```python
from build123d import *

# Parameters (mm, degrees)
SKETCH1_R           = 31.5
SKETCH1_R_2         = 4
SKETCH1_R_3         = 5.1
SKETCH1_R_4         = 3.5
SKETCH1_R_5         = 3
SKETCH1_R_6         = 3.000009018
BOSS_EXTRUDE1_DEPTH = 10
SKETCH1_3_R         = 5.1
SKETCH1_3_R_2       = 3.5
SKETCH1_3_R_3       = 3
SKETCH1_3_R_4       = 2.5
SKETCH1_3_R_5       = 3.000009018
BOSS_EXTRUDE2_DEPTH = 2


with BuildPart() as part:
    # Sketch1 → Boss-Extrude1 (new body)
    with BuildSketch(Plane.XY):
        Circle(SKETCH1_R)
        Circle(SKETCH1_R_2, mode=Mode.SUBTRACT)
        with Locations((-19, 0)):
            Circle(SKETCH1_R_3, mode=Mode.SUBTRACT)
        with Locations((0, 19)):
            Circle(SKETCH1_R_3, mode=Mode.SUBTRACT)
        with Locations((-13.436536842, 13.433520674)):
            Circle(SKETCH1_R_4, mode=Mode.SUBTRACT)
        with Locations((19, 0)):
            Circle(SKETCH1_R_3, mode=Mode.SUBTRACT)
        with Locations((13.436536842, -13.433520674)):
            Circle(SKETCH1_R_4, mode=Mode.SUBTRACT)
        with Locations((0, -19)):
            Circle(SKETCH1_R_3, mode=Mode.SUBTRACT)
        with Locations((8.124653839, 25)):
            Circle(SKETCH1_R_5, mode=Mode.SUBTRACT)
        with Locations((-9.156294472, -23.262894737)):
            Circle(SKETCH1_R_6, mode=Mode.SUBTRACT)
    extrude(amount=BOSS_EXTRUDE1_DEPTH)

    # Sketch1_3 → Boss-Extrude2 (add)
    with BuildSketch(Plane.XY):
        with Locations((19, 0)):
            Circle(SKETCH1_3_R)
        with Locations((19, 0)):
            Circle(SKETCH1_3_R_2, mode=Mode.SUBTRACT)
        with Locations((0, 19)):
            Circle(SKETCH1_3_R)
        with Locations((0, 19)):
            Circle(SKETCH1_3_R_2, mode=Mode.SUBTRACT)
        with Locations((13.436536842, -13.433520674)):
            Circle(SKETCH1_3_R_2)
        with Locations((13.436536842, -13.433520674)):
            Circle(SKETCH1_3_R_3, mode=Mode.SUBTRACT)
        with Locations((-13.436536842, 13.433520674)):
            Circle(SKETCH1_3_R_2)
        with Locations((-13.436536842, 13.433520674)):
            Circle(SKETCH1_3_R_3, mode=Mode.SUBTRACT)
        with Locations((0, -19)):
            Circle(SKETCH1_3_R)
        with Locations((0, -19)):
            Circle(SKETCH1_3_R_2, mode=Mode.SUBTRACT)
        with Locations((-19, 0)):
            Circle(SKETCH1_3_R)
        with Locations((-19, 0)):
            Circle(SKETCH1_3_R_2, mode=Mode.SUBTRACT)
        with Locations((8.124653839, 25)):
            Circle(SKETCH1_3_R_3)
        with Locations((8.124653839, 25)):
            Circle(SKETCH1_3_R_4, mode=Mode.SUBTRACT)
        with Locations((-9.156294472, -23.262894737)):
            Circle(SKETCH1_3_R_5)
        with Locations((-9.156294472, -23.262894737)):
            Circle(SKETCH1_3_R_4, mode=Mode.SUBTRACT)
    extrude(amount=BOSS_EXTRUDE2_DEPTH)


solid = part.part
```
Could you check a few things on this model? Use its own coordinates, in mm. A direction names the side the tool comes from. Give positions to 0.01 mm unless a question says otherwise; leave off trailing zeros. Write each loop counter-clockwise with the first axis right and the second up, starting at its lowest first coordinate (ties: lowest second). Pieces come first, ordered by that corner, then holes. Notation, with made-up numbers: (9.25, 46.25) - (16.25, 46.25) arc R28 cw to (16.25, 84.25) - close; hole circle Ø8 at (-34.5, -39). An arc over 180 degrees is marked (long way). One line per item, written item: value. Start each with the question number.
Item 1: Imagine slicing it at B-B, the plane z = 9. Give the number of separate pieces and of enclosed holes in the cut face, and give its area (3 significant figures).
Item 2: I'm going to push flat-ended pins straight in: pin 1 (3 mm diameter, centred on x = 2.5, z = 4.5, fed in from +Y); pin 2 (3.5 mm diameter, centred on x = -14, y = 15, fed in from +Z); pin 3 (13.5 mm diameter, centred on x = 0, y = 19, fed in from -Z); pin 4 (1 mm diameter, centred on y = 25, z = 5, fed in from +X). Where does each tip first touch, or does it pass through?
Item 3: Which directions (+Z, -Z, +X, -X, +Y, -Y) give clear straight access to the entire face, cutting with the end or side of a thin tool? Please do faces 1 (the face through (7.474, 22.071, 5.944)), 2 (the face through (-9.482, -20.784, 0.986)).
Item 4: Imagine slicing it at A-A, the plane x = 0. List the corners of the cut face in (y, z) for me, and give its area (3 significant figures).
Item 5: If we mould it in two halves opening along Y, with no side actions, what happens to faces 3 (the face through (-16.434, 13.565, 0.986)), 4 (the face through (7, 0, 10)), 5 (the face through (-4.101, 31.232, 4.93))? For each: +Y half, -Y half, draft (parallel to the pull), parting line (faces both ways), or undercut.
Item 6: Imagine slicing it at C-C, the plane y = 19. List the corners of the cut face in (x, z) for me, and give its area (3 significant figures).
Item 7: Please list where these lines run through material, in increasing order: line 1 (Y direction, x = 0, z = 9); line 2 (Y direction, x = 0, z = 1.3); line 3 (X direction, y = -15.5, z = 5). Write a range as from..to.
Geometry says:
1. separate pieces: 1
1. enclosed holes: 9
1. area: 2,610 mm^2
2. pin 1: y = 31.48
2. pin 2: z = 2
2. pin 3: z = 0
2. pin 4: x = 19.8
3. face 1: +Z
3. face 2: +Z, -Z
4. outline: (-31.5, 0) - (-22.5, 0) - (-22.5, 2) - (-24.1, 2) - (-24.1, 10) - (-31.5, 10) - close; (-15.5, 0) - (-4, 0) - (-4, 10) - (-13.9, 10) - (-13.9, 2) - (-15.5, 2) - close; (4, 0) - (15.5, 0) - (15.5, 2) - (13.9, 2) - (13.9, 10) - (4, 10) - close; (22.5, 0) - (31.5, 0) - (31.5, 10) - (24.1, 10) - (24.1, 2) - (22.5, 2) - close
4. area: 359 mm^2
5. face 3: undercut
5. face 4: draft
5. face 5: parting line
6. outline: (-25.12, 0) - (-3.5, 0) - (-3.5, 2) - (-5.1, 2) - (-5.1, 10) - (-25.12, 10) - close; (3.5, 0) - (25.12, 0) - (25.12, 10) - (5.1, 10) - (5.1, 2) - (3.5, 2) - close
6. area: 407 mm^2
7. line 1: -31.5..-24.1, -13.9..-4, 4..13.9, 24.1..31.5
7. line 2: -31.5..-22.5, -15.5..-4, 4..15.5, 22.5..31.5
7. line 3: -27.42..-3.71, 3.71..10.61, 16.26..27.42
